```python
from build123d import *

# Parameters (mm, degrees)
SKETCH2_W           = 20.32
SKETCH2_H           = 127
BOSS_EXTRUDE1_DEPTH = 2.999994
BOSS_EXTRUDE2_DEPTH = 2.999994
SKETCH6_R           = 2.54
CUT_EXTRUDE2_DEPTH  = 171.130289375


with BuildPart() as part:
    # Sketch2 → Boss-Extrude1 (new body)
    with BuildSketch(Plane(origin=(0, 0, 0), x_dir=(1, 0, 0), z_dir=(0, 1, 0))):
        Rectangle(SKETCH2_W, SKETCH2_H)
    extrude(amount=BOSS_EXTRUDE1_DEPTH)

    # Sketch4 → Boss-Extrude2 (add)
    with BuildSketch(Plane(origin=(0, 10.859139551, 61.58524071), x_dir=(1, 0, 0), z_dir=(0, 0.173648178, 0.984807753))):
        Polygon((10.16, -8.072241932), (-10.16, -8.072241932), (-10.16, -135.072241932), (0, -135.072241932), (10.16, -135.072241932), align=None)
    boss_extrude2 = extrude(amount=-BOSS_EXTRUDE2_DEPTH)

    # Mirror1: Boss-Extrude2 across plane
    add(boss_extrude2.mirror(Plane.XY))

    # Sketch6 → Cut-Extrude2 (cut, through all)
    with BuildSketch(Plane.XY.offset(85.09)):
        with Locations((0, -114.54105152)):
            Circle(SKETCH6_R)
    extrude(amount=-CUT_EXTRUDE2_DEPTH, mode=Mode.SUBTRACT)


solid = part.part
```
Part model, mm, in its own coordinate system. A direction names the side the tool comes from. Coordinates: 2 decimals unless noted, no trailing zeros. Order: outer loops, then holes, each group sorted by start corner. A loop starts at its lowest first (then second) coordinate and runs counter-clockwise, first axis right, second up. Notation, with made-up numbers: (0.5, 43.25) - (31.5, 43.25) arc R22 cw to (31.5, 67.25) - close; hole circle Ø10 at (-20, -34.5). An arc over 180 degrees is marked (long way). Return JSON: item names as keys, results as strings. Group by question number.
Item 1: Cut at C-C (z = -37). List the corners of the cut face in (x, y).
Item 2: Cut at A-A (x = -6.5). List the corners of the cut face in (y, z), plus the area to 3 significant figures.
Item 3: Pull direction Y, two halves, no side cores. Call faces 1 (the face through (-0.14, -60.23, -74.12)), 2 (the face through (10.16, 2, 10)), 3 (the face through (0, -112, 82)), 4 (the face through (-0.14, -60.48, 71.12)): pulls with the +Y half, pulls with the -Y half, needs draft (parallel to the pull), parting line crosses it, or undercut.
Item 4: Cut at D-D (z = -75). List the corners of the cut face in (x, y), plus the area to 3 significant figures.
Item 5: Drill centre lines: probe 1 along Y at (x, z) = (9.25, 30.5); probe 2 along Z at (x, y) = (-3.75, -27); probe 3 along Z at (x, y) = (-6.75, -61). Where is each one in solid material? Low to high. Write a range as from..to.
Item 6: Pin check, flat tips, straight feed: pin 1 (3 mm diameter, centred on x = 1, z = -15, fed in from -Y); pin 2 (3.5 mm diameter, centred on x = 2.5, y = 1, fed in from -Z); pin 3 (4 mm diameter, centred on x = 0, y = -114.54, fed in from +Z); pin 4 (8 mm diameter, centred on x = -3, y = -66, fed in from -Z). Stop position of each tip, or through.
Item 7: Which spindle directions (+Z, -Z, +X, -X, +Y, -Y) get a long thin tool onto all of the face, cutting with end or side? Do faces 5 (the face through (-0.14, -60.48, -71.12)), 6 (the face through (-0.14, -60.23, 74.12)). Say none if no direction does.
Item 8: Cut at B-B (y = -84.5). List the corners of the cut face in (x, z), plus the area to 3 significant figures.
Check values:
{
 "1": {"outline": "(-10.16, 0) - (10.16, 0) - (10.16, 3) - (-10.16, 3) - close"},
 "2": {"outline": "(-122.68, -82.09) - (-122.16, -85.04) - (0, -63.5) - (3, -63.5) - (3, 63.5) - (0, 63.5) - (-122.16, 85.04) - (-122.68, 82.09) - (0, 60.45) - (0, -60.45) - close", "area": "1,130 mm2"},
 "3": {"face 1": "pulls with the +Y half", "face 2": "needs draft", "face 3": "undercut", "face 4": "pulls with the -Y half"},
 "4": {"outline": "(-10.16, -82.5) - (10.16, -82.5) - (10.16, -65.22) - (-10.16, -65.22) - close", "area": "351 mm2"},
 "5": {"probe 1": "y = 0..3", "probe 2": "z = -68.26..-65.21, 65.21..68.26", "probe 3": "z = -74.26..-71.21, 71.21..74.26"},
 "6": {"pin 1": "stops at y = 0", "pin 2": "stops at z = -63.63", "pin 3": "passes through", "pin 4": "stops at z = -75.84"},
 "7": {"face 5": "+X, -X, -Y", "face 6": "+Z, +X, -X, +Y"},
 "8": {"outline": "(-10.16, -78.4) - (10.16, -78.4) - (10.16, -75.35) - (-10.16, -75.35) - close; (-10.16, 75.35) - (10.16, 75.35) - (10.16, 78.4) - (-10.16, 78.4) - close", "area": "124 mm2"}
}
